```python
from build123d import *

# Parameters (mm, degrees)
SKETCH_1_W          = 40
SKETCH_1_H          = 40
EXTRUDE_1_DEPTH     = 6
SKETCH_1_3_W        = 5
SKETCH_1_3_H        = 40
SKETCH_1_3_W_2      = 10
EXTRUDE_2_DEPTH     = 34
CUT_EXTRUDE_1_DEPTH = 20
CUT_EXTRUDE_2_REACH = 50.99
SKETCH_4_R          = 2.5
SKETCH_5_R          = 1.5
CUT_EXTRUDE_3_DEPTH = 5
CUT_EXTRUDE_4_REACH = 51.558
SKETCH_7_R          = 1.5
CUT_EXTRUDE_5_REACH = 58.178
SKETCH_8_R          = 11.75
CUT_EXTRUDE_6_REACH = 58.178
SKETCH_9_R          = 11
CHAMFER_1_SIZE      = 0.5
CHAMFER_2_SIZE      = 0.3
CHAMFER_3_SIZE      = 0.5
CHAMFER_4_SIZE      = 0.5
CHAMFER_5_SIZE      = 0.5
CHAMFER_6_SIZE      = 0.5
CHAMFER_7_SIZE      = 0.4
CHAMFER_8_SIZE      = 0.4
CHAMFER_9_SIZE      = 0.5
CHAMFER_10_SIZE     = 0.5
CHAMFER_11_SIZE     = 0.4
CHAMFER_12_SIZE     = 0.4


# Read off the part's stored shape, not the designer's step: 高级异型孔6, 高级异型孔7, 镜向4
with BuildPart() as part:
    # 草图1 → 凸台-拉伸1 (new body)
    with BuildSketch(Plane(origin=(0, 0, 0), x_dir=(1, 0, 0), z_dir=(0, 1, 0))):
        Rectangle(SKETCH_1_W, SKETCH_1_H)
    extrude(amount=EXTRUDE_1_DEPTH)

    # 草图1<3> → 凸台-拉伸2 (add)
    with BuildSketch(Plane(origin=(0, 0, 0), x_dir=(1, 0, 0), z_dir=(0, 1, 0))):
        with Locations((-17.5, 0)):
            Rectangle(SKETCH_1_3_W, SKETCH_1_3_H)
        with Locations((15, 0)):
            Rectangle(SKETCH_1_3_W_2, SKETCH_1_3_H)
    extrude(amount=-EXTRUDE_2_DEPTH)

    # 草图3 → 切除-拉伸1 (cut, symmetric)
    with BuildSketch(Plane(origin=(0, 0, 0), x_dir=(0, 0, -1), z_dir=(1, 0, 0))):
        Polygon((20, -28), (11.43111196, -34), (20, -34), align=None)
        Polygon((-20, -34), (-20, -28), (-11.43111196, -34), align=None)
    extrude(amount=CUT_EXTRUDE_1_DEPTH, both=True, mode=Mode.SUBTRACT)

    # 草图4 → 切除-拉伸2 (cut, up to next)
    with BuildSketch(Plane(origin=(0, 6, 0), x_dir=(1, 0, 0), z_dir=(0, 1, 0)), mode=Mode.PRIVATE) as cut_extrude_2_sk1:
        with Locations(Location((0, -10, 0), (0, 0, 270))):
            Circle(SKETCH_4_R)
    cut_extrude_2_tool1 = extrude(cut_extrude_2_sk1.sketch, amount=-CUT_EXTRUDE_2_REACH, mode=Mode.PRIVATE) & part.part
    # 草图4 → 切除-拉伸2 (cut, up to next)
    with BuildSketch(Plane(origin=(0, 6, 0), x_dir=(1, 0, 0), z_dir=(0, 1, 0)), mode=Mode.PRIVATE) as cut_extrude_2_sk2:
        with Locations(Location((0, 10, 0), (0, 0, 270))):
            Circle(SKETCH_4_R)
    cut_extrude_2_tool2 = extrude(cut_extrude_2_sk2.sketch, amount=-CUT_EXTRUDE_2_REACH, mode=Mode.PRIVATE) & part.part
    add(cut_extrude_2_tool1.solids().sort_by_distance((0, 6, 10))[0], mode=Mode.SUBTRACT)
    add(cut_extrude_2_tool2.solids().sort_by_distance((0, 6, -10))[0], mode=Mode.SUBTRACT)

    # 草图5 → 切除-拉伸3 (cut)
    with BuildSketch(Plane(origin=(-15, 0, 0), x_dir=(0, 0, -1), z_dir=(1, 0, 0))):
        with Locations((-10.61, -3.39)):
            Circle(SKETCH_5_R)
        with Locations((-10.61, -24.6)):
            Circle(SKETCH_5_R)
        with Locations((10.6, -24.6)):
            Circle(SKETCH_5_R)
        with Locations((10.6, -3.39)):
            Circle(SKETCH_5_R)
    extrude(amount=-CUT_EXTRUDE_3_DEPTH, mode=Mode.SUBTRACT)

    # 草图7 → 切除-拉伸4 (cut, up to next)
    with BuildSketch(Plane.ZY.offset(-10), mode=Mode.PRIVATE) as cut_extrude_4_sk1:
        with Locations((9.9, -4.39)):
            Circle(SKETCH_7_R)
    cut_extrude_4_tool1 = extrude(cut_extrude_4_sk1.sketch, amount=-CUT_EXTRUDE_4_REACH, mode=Mode.PRIVATE) & part.part
    # 草图7 → 切除-拉伸4 (cut, up to next)
    with BuildSketch(Plane.ZY.offset(-10), mode=Mode.PRIVATE) as cut_extrude_4_sk2:
        with Locations((9.9, -24.19)):
            Circle(SKETCH_7_R)
    cut_extrude_4_tool2 = extrude(cut_extrude_4_sk2.sketch, amount=-CUT_EXTRUDE_4_REACH, mode=Mode.PRIVATE) & part.part
    # 草图7 → 切除-拉伸4 (cut, up to next)
    with BuildSketch(Plane.ZY.offset(-10), mode=Mode.PRIVATE) as cut_extrude_4_sk3:
        with Locations((-9.9, -24.19)):
            Circle(SKETCH_7_R)
    cut_extrude_4_tool3 = extrude(cut_extrude_4_sk3.sketch, amount=-CUT_EXTRUDE_4_REACH, mode=Mode.PRIVATE) & part.part
    # 草图7 → 切除-拉伸4 (cut, up to next)
    with BuildSketch(Plane.ZY.offset(-10), mode=Mode.PRIVATE) as cut_extrude_4_sk4:
        with Locations((-9.9, -4.39)):
            Circle(SKETCH_7_R)
    cut_extrude_4_tool4 = extrude(cut_extrude_4_sk4.sketch, amount=-CUT_EXTRUDE_4_REACH, mode=Mode.PRIVATE) & part.part
    add(cut_extrude_4_tool1.solids().sort_by_distance((10, -4.39, 9.9))[0], mode=Mode.SUBTRACT)
    add(cut_extrude_4_tool2.solids().sort_by_distance((10, -24.19, 9.9))[0], mode=Mode.SUBTRACT)
    add(cut_extrude_4_tool3.solids().sort_by_distance((10, -24.19, -9.9))[0], mode=Mode.SUBTRACT)
    add(cut_extrude_4_tool4.solids().sort_by_distance((10, -4.39, -9.9))[0], mode=Mode.SUBTRACT)

    # 草图8 → 切除-拉伸5 (cut, up to next)
    with BuildSketch(Plane(origin=(20, 0, 0), x_dir=(0, 0, -1), z_dir=(1, 0, 0)), mode=Mode.PRIVATE) as cut_extrude_5_sk1:
        with Locations((0, -14)):
            Circle(SKETCH_8_R)
    cut_extrude_5_tool1 = extrude(cut_extrude_5_sk1.sketch, amount=-CUT_EXTRUDE_5_REACH, mode=Mode.PRIVATE) & part.part
    add(cut_extrude_5_tool1.solids().sort_by_distance((20, -14, 0))[0], mode=Mode.SUBTRACT)

    # 草图9 → 切除-拉伸6 (cut, up to next)
    with BuildSketch(Plane.ZY.offset(20), mode=Mode.PRIVATE) as cut_extrude_6_sk1:
        with Locations((0, -14)):
            Circle(SKETCH_9_R)
    cut_extrude_6_tool1 = extrude(cut_extrude_6_sk1.sketch, amount=-CUT_EXTRUDE_6_REACH, mode=Mode.PRIVATE) & part.part
    add(cut_extrude_6_tool1.solids().sort_by_distance((-20, -14, 0))[0], mode=Mode.SUBTRACT)

    # 倒角1
    chamfer_1_edges = [part.edges().sort_by_distance(p)[0] for p in [
        (20, -14, 11.75),
    ]]
    chamfer(chamfer_1_edges, length=CHAMFER_1_SIZE)

    # 倒角2
    chamfer_2_edges = [part.edges().sort_by_distance(p)[0] for p in [
        (10, -14, 11.75),
    ]]
    chamfer(chamfer_2_edges, length=CHAMFER_2_SIZE)

    # 倒角3
    chamfer_3_edges = [part.edges().sort_by_distance(p)[0] for p in [
        (-20, -14, -11),
    ]]
    chamfer(chamfer_3_edges, length=CHAMFER_3_SIZE)

    # 倒角4
    chamfer_4_edges = [part.edges().sort_by_distance(p)[0] for p in [
        (-15, -14, -11),
    ]]
    chamfer(chamfer_4_edges, length=CHAMFER_4_SIZE)

    # 高级异型孔6 outline → 高级异型孔6 (revolve, cut)
    with BuildSketch(Plane(origin=(-17.29366154, -25.01, 0), x_dir=(1, 0, 0), z_dir=(0, -1, 0))):
        Polygon((0, -20), (1.250000655, -20), (1.25, -10), (0.81997305, -9.741613741), (0, -9.741613741), align=None)
    revolve(axis=Axis((-17.29366154, -25.01, 0), (0, 0, 1)), mode=Mode.SUBTRACT)

    # Other 6 2 outline → Other 6 2 (revolve, cut)
    with BuildSketch(Plane(origin=(-17.5, 0.99, 0), x_dir=(1, 0, 0), z_dir=(0, -1, 0))):
        Polygon((1.25, -20), (1.25, -10), (0, -9.248924226), (0, -20), align=None)
    revolve(axis=Axis((-17.5, 0.99, 0), (0, 0, 1)), mode=Mode.SUBTRACT)

    # 高级异型孔7 outline → 高级异型孔7 (revolve, cut)
    with BuildSketch(Plane(origin=(15, 0.99, 0), x_dir=(1, 0, 0), z_dir=(0, -1, 0))):
        Polygon((2, -20), (2, -10), (0, -8.798278762), (0, -20), align=None)
    revolve(axis=Axis((15, 0.99, 0), (0, 0, 1)), mode=Mode.SUBTRACT)

    # Other 7 2 outline → Other 7 2 (revolve, cut)
    with BuildSketch(Plane(origin=(15.20633846, -25.01, 0), x_dir=(1, 0, 0), z_dir=(0, -1, 0))):
        Polygon((2, -20), (2, -10), (0.412753929, -9.046286343), (0, -9.046286343), (0, -20), align=None)
    revolve(axis=Axis((15.20633846, -25.01, 0), (0, 0, 1)), mode=Mode.SUBTRACT)

    # 倒角5
    chamfer_5_edges = [part.edges().sort_by_distance(p)[0] for p in [
        (13, 0.99, -20),
    ]]
    chamfer(chamfer_5_edges, length=CHAMFER_5_SIZE)

    # 倒角6
    chamfer_6_edges = [part.edges().sort_by_distance(p)[0] for p in [
        (13.20633846, -25.01, -20),
    ]]
    chamfer(chamfer_6_edges, length=CHAMFER_6_SIZE)

    # 倒角7
    chamfer_7_edges = [part.edges().sort_by_distance(p)[0] for p in [
        (-18.543662195, -25.01, -20),
    ]]
    chamfer(chamfer_7_edges, length=CHAMFER_7_SIZE)

    # 倒角8
    chamfer_8_edges = [part.edges().sort_by_distance(p)[0] for p in [
        (-18.75, 0.99, -20),
    ]]
    chamfer(chamfer_8_edges, length=CHAMFER_8_SIZE)

    # 镜向4 outline → 镜向4 (revolve, cut)
    with BuildSketch(Plane(origin=(-17.29366154, -25.01, 0), x_dir=(1, 0, 0), z_dir=(0, -1, 0))):
        Polygon((0.807641167, 9.734203998), (1.25, 10), (1.25, 20), (0, 20), (0, 9.734203998), align=None)
    revolve(axis=Axis((-17.29366154, -25.01, 0), (0, 0, 1)), mode=Mode.SUBTRACT)

    # Mirror 4 2 outline → Mirror 4 2 (revolve, cut)
    with BuildSketch(Plane(origin=(-17.5, 0.99, 0), x_dir=(1, 0, 0), z_dir=(0, -1, 0))):
        Polygon((0, 9.248924226), (1.25, 10), (1.25, 20), (0, 20), align=None)
    revolve(axis=Axis((-17.5, 0.99, 0), (0, 0, 1)), mode=Mode.SUBTRACT)

    # Mirror 4 3 outline → Mirror 4 3 (revolve, cut)
    with BuildSketch(Plane(origin=(15, 0.99, 0), x_dir=(1, 0, 0), z_dir=(0, -1, 0))):
        Polygon((0, 8.798278762), (2, 10), (2, 20), (0, 20), align=None)
    revolve(axis=Axis((15, 0.99, 0), (0, 0, 1)), mode=Mode.SUBTRACT)

    # Mirror 4 4 outline → Mirror 4 4 (revolve, cut)
    with BuildSketch(Plane(origin=(15.20633846, -25.01, 0), x_dir=(1, 0, 0), z_dir=(0, -1, 0))):
        Polygon((0.412753929, 9.046286343), (2, 10), (2, 20), (0, 20), (0, 9.046286343), align=None)
    revolve(axis=Axis((15.20633846, -25.01, 0), (0, 0, 1)), mode=Mode.SUBTRACT)

    # 倒角9
    chamfer_9_edges = [part.edges().sort_by_distance(p)[0] for p in [
        (13.20633846, -25.01, 20),
    ]]
    chamfer(chamfer_9_edges, length=CHAMFER_9_SIZE)

    # 倒角10
    chamfer_10_edges = [part.edges().sort_by_distance(p)[0] for p in [
        (13, 0.99, 20),
    ]]
    chamfer(chamfer_10_edges, length=CHAMFER_10_SIZE)

    # 倒角11
    chamfer_11_edges = [part.edges().sort_by_distance(p)[0] for p in [
        (-18.54366154, -25.01, 20),
    ]]
    chamfer(chamfer_11_edges, length=CHAMFER_11_SIZE)

    # 倒角12
    chamfer_12_edges = [part.edges().sort_by_distance(p)[0] for p in [
        (-18.75, 0.99, 20),
    ]]
    chamfer(chamfer_12_edges, length=CHAMFER_12_SIZE)


solid = part.part
```
The model under review builds one solid part; all positions refer to its coordinate system, in mm. A direction names the side the tool comes from. Give positions to 0.01 mm unless a question says otherwise; leave off trailing zeros. Order: outer loops, then holes, each group sorted by start corner. A loop starts at its lowest first (then second) coordinate and runs counter-clockwise, first axis right, second up. Notation, with made-up numbers: (43.5, 10) - (75.5, 10) arc R5 ccw to (75.5, 15) - close; hole circle Ø5 at (-22.75, 89). An arc over 180 degrees is marked (long way). Use CSV: the item, a comma, the result in double quotes. Start each with the question number.
Q1. Clearance check with flat-ended pins moving along their axes: pin 1 Ø4 at (x, z) = (0, 10) entering from -Y (1 decimal); pin 2 Ø2.5 at (y, z) = (-24.19, -9.9) entering from +X; pin 3 Ø2 at (x, y) = (-17.5, 0.99) entering from +Z; pin 4 Ø2.5 at (y, z) = (-3.39, 10.61) entering from -X. State where each tip first meets the part, or that it passes through.
Q2. Tool access review of faces 1 (the cylindrical face through (14.93, -23.74, -8.47)), 2 (the cylindrical face through (-17.46, -23.59, -9.49)), 3 (the cylindrical face through (-17.56, -26.23, -15.8)), 4 (the flat face through (-3, 0, 0)): name each direction out of +Z, -Z, +X, -X, +Y, -Y from which nothing blocks a thin tool from reaching the whole face with its end or side.
Q3. We need section A-A, the plane z = 0. Write out the cut boundary in (x, y), and give its area (3 significant figures).
Q4. We need section C-C, the plane z = -16.5. Write out the cut boundary in (x, y).
Q5. The part is to be moulded in two halves that separate along Y. For faces 5 (the cylindrical face through (-17.56, -26.23, 15.93)), 6 (the flat face through (-20, -5, -9)), 7 (the flat face through (-18, -34, 0)), 8 (the cylindrical face through (13.526, 2.342, -14.683)), say which applies: +Y half, -Y half, draft (parallel to the pull), parting line (faces both ways), or undercut.
Q6. We need section B-B, the plane y = -14. Write out the cut boundary in (x, z).
Q7. To check wall thickness, follow line 1 along X through (y, z) = (-25, 14); line 2 along X through (y, z) = (-29, -11); line 3 along Y through (x, z) = (18.25, -9.9). State the ranges of each line that lie inside material, in increasing order. Write a range as [from, to].
Q8. We need section D-D, the plane x = -5.5. Write out the cut boundary in (y, z).
Outcome:
1,pin 1,"passes through"
1,pin 2,"stops at x = -15"
1,pin 3,"stops at z = 9.85"
1,pin 4,"stops at x = 10"
2,face 1,"+X"
2,face 2,"-X"
2,face 3,"-Z"
2,face 4,"+Z, -Z, -Y"
3,outline,"(-20, -34) - (-15, -34) - (-15, -25.5) - (-15.5, -25) - (-19.5, -25) - (-20, -25.5) - close; (-20, -2.5) - (-19.5, -3) - (-15.5, -3) - (-15, -2.5) - (-15, 0) - (10, 0) - (10, -1.95) - (10.3, -2.25) - (19.5, -2.25) - (20, -1.75) - (20, 6) - (-20, 6) - close; (10, -34) - (20, -34) - (20, -26.25) - (19.5, -25.75) - (10.3, -25.75) - (10, -26.05) - close"
3,area,"404 mm^2"
4,outline,"(-20, -30.45) - (-15, -30.45) - (-15, 0) - (10, 0) - (10, -30.45) - (20, -30.45) - (20, 6) - (-20, 6) - close; hole circle Ø2.5 at (-17.5, 0.99); hole circle Ø2.5 at (-17.29, -25.01); hole circle Ø4 at (15, 0.99); hole circle Ø4 at (15.21, -25.01)"
5,face 5,"undercut"
5,face 6,"draft"
5,face 7,"-Y half"
5,face 8,"undercut"
6,outline,"(-20, -20) - (-15, -20) - (-15, -11.5) - (-15.5, -11) - (-19.5, -11) - (-20, -11.5) - close; (-20, 11.5) - (-19.5, 11) - (-15.5, 11) - (-15, 11.5) - (-15, 20) - (-20, 20) - close; (10, -20) - (20, -20) - (20, -12.25) - (19.5, -11.75) - (10.3, -11.75) - (10, -12.05) - close; (10, 12.05) - (10.3, 11.75) - (19.5, 11.75) - (20, 12.25) - (20, 20) - (10, 20) - close"
7,line 1,"x = [-20, -18.54], [-16.04, -15], [10, 13.21], [17.21, 20]"
7,line 2,"x = [-20, -15], [10, 20]"
7,line 3,"y = [-34, -25.69], [-22.69, -20.33], [-7.67, -5.89], [-2.89, 6]"
8,outline,"(0, -20) - (6, -20) - (6, 20) - (0, 20) - close"
